from build123d import *

# Parameters (mm, degrees)
SKETCH1_W                 = 57.15
SKETCH1_H                 = 5.08
BOSS_EXTRUDE1_DEPTH       = 152.4
CUT_EXTRUDE1_DEPTH        = 1
SKETCH3_W                 = 57.15
SKETCH3_H                 = 5.08
BOSS_EXTRUDE2_DEPTH       = 12.7
SKETCH4_R                 = 2.25
CUT_EXTRUDE2_DEPTH        = 12.7
SKETCH5_R                 = 0.889
CUT_EXTRUDE3_DEPTH        = 156.961081764
SKETCH6_W                 = 57.15
SKETCH6_H                 = 4.08
BOSS_EXTRUDE3_DEPTH       = 5
SKETCH7_R                 = 0.889
CUT_EXTRUDE4_DEPTH        = 161.850424386
LPATTERN1_COUNT           = 6
LPATTERN1_PITCH           = 25
LPATTERN1_COPY_1_SKETCH_R = 0.889
LPATTERN1_COPY_1_DEPTH    = 161.850424386
LPATTERN1_COPY_2_SKETCH_R = 0.889
LPATTERN1_COPY_2_DEPTH    = 161.850424386
LPATTERN1_COPY_3_SKETCH_R = 0.889
LPATTERN1_COPY_3_DEPTH    = 161.850424386
LPATTERN1_COPY_4_SKETCH_R = 0.889
LPATTERN1_COPY_4_DEPTH    = 161.850424386
LPATTERN1_COPY_5_SKETCH_R = 0.889
LPATTERN1_COPY_5_DEPTH    = 161.850424386


with BuildPart() as part:
    # Sketch1 → Boss-Extrude1 (new body)
    with BuildSketch(Plane(origin=(0, 0, 0), x_dir=(1, 0, 0), z_dir=(0, 1, 0))):
        Rectangle(SKETCH1_W, SKETCH1_H)
    extrude(amount=-BOSS_EXTRUDE1_DEPTH)

    # Sketch2 → Cut-Extrude1 (cut)
    with BuildSketch(Plane.XY.offset(2.54)):
        Polygon((-5, -152.4), (-5, -53.9), (5, -53.9), (5, -152.4), (28.575, -152.4), (28.575, -14.9), (-28.575, -14.9), (-28.575, -152.4), align=None)
    extrude(amount=-CUT_EXTRUDE1_DEPTH, mode=Mode.SUBTRACT)

    # Sketch3 → Boss-Extrude2 (add)
    with BuildSketch(Plane(origin=(0, 0, -2.54), x_dir=(-1, 0, 0), z_dir=(0, 0, -1))):
        with Locations((0, -2.54)):
            Rectangle(SKETCH3_W, SKETCH3_H)
    extrude(amount=BOSS_EXTRUDE2_DEPTH)

    # Sketch4 → Cut-Extrude2 (cut)
    with BuildSketch(Plane(origin=(0, 0, 0), x_dir=(1, 0, 0), z_dir=(0, 1, 0))):
        with Locations(Location((0, 10.16, 0), (0, 0, 270))):
            Circle(SKETCH4_R)
    extrude(amount=-CUT_EXTRUDE2_DEPTH, mode=Mode.SUBTRACT)

    # Sketch5 → Cut-Extrude3 (cut, through all)
    with BuildSketch(Plane.XY.offset(1.54)):
        with Locations((-19, -19.15)):
            Circle(SKETCH5_R)
        with Locations((19, -19.15)):
            Circle(SKETCH5_R)
        with Locations((-19, -148.65)):
            Circle(SKETCH5_R)
        with Locations((19, -148.65)):
            Circle(SKETCH5_R)
    extrude(amount=-CUT_EXTRUDE3_DEPTH, mode=Mode.SUBTRACT)

    # Sketch6 → Boss-Extrude3 (add)
    with BuildSketch(Plane.XZ.offset(152.4)):
        with Locations((0, -0.5)):
            Rectangle(SKETCH6_W, SKETCH6_H)
    extrude(amount=BOSS_EXTRUDE3_DEPTH)

    # Sketch7 → Cut-Extrude4 (cut, through all)
    with BuildSketch(Plane.XY.offset(1.54)):
        with Locations((-25.575, -154.4)):
            Circle(SKETCH7_R)
    cut_extrude4 = extrude(amount=-CUT_EXTRUDE4_DEPTH, mode=Mode.SUBTRACT)

    # Mirror1: Cut-Extrude4 across plane
    add(cut_extrude4.mirror(Plane(origin=(0, 0, 0), x_dir=(0, 0, 1), z_dir=(1, 0, 0))), mode=Mode.SUBTRACT)

    # LPattern1: Cut-Extrude4 ×6
    with Locations(*[(0, i * LPATTERN1_PITCH, 0) for i in range(1, LPATTERN1_COUNT)]):
        add(cut_extrude4, mode=Mode.SUBTRACT)

    # LPattern1 copy 1 sketch → LPattern1 copy 1 (cut, through all)
    with BuildSketch(Plane(origin=(0, 25, 1.54), x_dir=(-1, 0, 0), z_dir=(0, 0, 1))):
        with Locations((-25.575, 154.4)):
            Circle(LPATTERN1_COPY_1_SKETCH_R)
    extrude(amount=-LPATTERN1_COPY_1_DEPTH, mode=Mode.SUBTRACT)

    # LPattern1 copy 2 sketch → LPattern1 copy 2 (cut, through all)
    with BuildSketch(Plane(origin=(0, 50, 1.54), x_dir=(-1, 0, 0), z_dir=(0, 0, 1))):
        with Locations((-25.575, 154.4)):
            Circle(LPATTERN1_COPY_2_SKETCH_R)
    extrude(amount=-LPATTERN1_COPY_2_DEPTH, mode=Mode.SUBTRACT)

    # LPattern1 copy 3 sketch → LPattern1 copy 3 (cut, through all)
    with BuildSketch(Plane(origin=(0, 75, 1.54), x_dir=(-1, 0, 0), z_dir=(0, 0, 1))):
        with Locations((-25.575, 154.4)):
            Circle(LPATTERN1_COPY_3_SKETCH_R)
    extrude(amount=-LPATTERN1_COPY_3_DEPTH, mode=Mode.SUBTRACT)

    # LPattern1 copy 4 sketch → LPattern1 copy 4 (cut, through all)
    with BuildSketch(Plane(origin=(0, 100, 1.54), x_dir=(-1, 0, 0), z_dir=(0, 0, 1))):
        with Locations((-25.575, 154.4)):
            Circle(LPATTERN1_COPY_4_SKETCH_R)
    extrude(amount=-LPATTERN1_COPY_4_DEPTH, mode=Mode.SUBTRACT)

    # LPattern1 copy 5 sketch → LPattern1 copy 5 (cut, through all)
    with BuildSketch(Plane(origin=(0, 125, 1.54), x_dir=(-1, 0, 0), z_dir=(0, 0, 1))):
        with Locations((-25.575, 154.4)):
            Circle(LPATTERN1_COPY_5_SKETCH_R)
    extrude(amount=-LPATTERN1_COPY_5_DEPTH, mode=Mode.SUBTRACT)


solid = part.part
Verification items for the finished model (mm, model axes). Coordinates: 2 decimals unless noted, no trailing zeros. Order: outer loops, then holes, each group sorted by start corner. A loop starts at its lowest first (then second) coordinate and runs counter-clockwise, first axis right, second up. Notation, with made-up numbers: M -35,25.5 L -14,25.5 A15 ccw -14,48.5 Z; hole C -31,30.5 d11. An arc over 180 degrees is marked long. One line per item, written item: value. Start each with the question number.
Item 1: Sectioned sample at C-C on x = 22.5. Record the cut outline in (y, z).
Item 2: Sectioned sample at A-A on x = 0. Record the cut outline in (y, z), then the cut area to 3 significant figures.
Item 3: Depth check by flat-ended pin: P1, Ø1.6, axis at x = 25.575, y = -129.4, coming from the -Z side (3 decimals); P2, Ø2, axis at x = 25.575, y = -79.4, coming from the +Z side; P3, Ø1.5, axis at x = -22.5, z = -4, coming from the -Y side; P4, Ø3, axis at x = 25.575, y = -154.4, coming from the -Z side. Enter the tip coordinate at first touch or a pass-through.
Item 4: Sectioned sample at B-B on y = -144.5. Record the cut outline in (x, z) (3 decimals).
Item 5: Thickness scan on probe 1 along X at (y, z) = (-104.4, 0.3) (3 decimals); probe 2 along Y at (x, z) = (-19, -0.5); probe 3 along Z at (x, y) = (25.5, -87). Record the ranges inside material, lowest first.
Item 6: Mould release check, pull along Z, two halves, no side actions. Record for faces 1 (the flat face through (0, -5.08, -7)), 2 (the cylindrical face through (0.676, -2.504, -8.014)), 3 (the flat face through (0, -80, -2.54)): pulls with the +Z half, pulls with the -Z half, needs draft (parallel to the pull), parting line crosses it, or undercut.
Item 7: Sectioned sample at D-D on z = -5.75. Record the cut outline in (x, y) (3 decimals).
Calculated:
1. outline: M -157.4,-2.54 L -5.08,-2.54 L -5.08,-15.24 L 0,-15.24 L 0,2.54 L -14.9,2.54 L -14.9,1.54 L -157.4,1.54 Z
2. outline: M -157.4,-2.54 L -5.08,-2.54 L -5.08,-7.91 L 0,-7.91 L 0,2.54 L -14.9,2.54 L -14.9,1.54 L -53.9,1.54 L -53.9,2.54 L -152.4,2.54 L -152.4,1.54 L -157.4,1.54 Z; M -5.08,-15.24 L 0,-15.24 L 0,-12.41 L -5.08,-12.41 Z
2. area: 797 mm^2
3. P1: through
3. P2: z = 1.54
3. P3: y = -5.08
3. P4: z = -2.54
4. outline: M -28.575,-2.54 L 28.575,-2.54 L 28.575,1.54 L 5,1.54 L 5,2.54 L -5,2.54 L -5,1.54 L -28.575,1.54 Z
5. probe 1: -28.575 to -26.464, -24.686 to 24.686, 26.464 to 28.575
5. probe 2: -157.4 to -149.54, -147.76 to -20.04, -18.26 to 0
5. probe 3: -2.54 to 1.54
6. face 1: needs draft
6. face 2: undercut
6. face 3: pulls with the -Z half
7. outline: M -28.575,-5.08 L 28.575,-5.08 L 28.575,0 L -28.575,0 Z
